Work out the finished part from the listing and answer in its coordinate system (mm). Face numbers are marked on the shaded views. A direction names the side the tool comes from. Round coordinates to 2 decimals unless told otherwise and drop trailing zeros. Loops run counter-clockwise (first coordinate to the right, second up) from the corner with the lowest first, then second, coordinate; pieces in that order, holes last.
```python
from build123d import *

# Parameters (mm, degrees)
BOSS_EXTRUDE1_DEPTH     = 27.94
CUT_EXTRUDE1_DEPTH      = 48.739163168
CUT_EXTRUDE1_DEPTH_BACK = 48.739163168
SKETCH3_R               = 6.35
CUT_EXTRUDE2_DEPTH      = 48.73916328
CUT_EXTRUDE2_DEPTH_BACK = 24.13
SKETCH4_R               = 8.001
CUT_EXTRUDE3_REACH      = 61.268
CUT_EXTRUDE3_START      = 12.192
SKETCH5_W               = 45.72
SKETCH5_H               = 20.574
SKETCH6_W               = 10.668
SKETCH6_H               = 4.572
CUT_EXTRUDE4_DEPTH      = 2.54
SKETCH7_W               = 12.7
SKETCH7_H               = 11.938
CUT_EXTRUDE5_DEPTH      = 2.54
FILLET1_R               = 5.08
CUT_EXTRUDE6_START      = 3.048
SKETCH8_W               = 48.26
SKETCH8_H               = 23.114
CUT_EXTRUDE6_DEPTH      = 12.7


with BuildPart() as part:
    # Sketch2 → Boss-Extrude1 (new body)
    with BuildSketch(Plane.XY):
        with BuildLine():
            Line((29.21, -5.08), (29.21, -25.4))
            Line((29.21, -25.4), (19.431, -25.4))
            ThreePointArc((19.431, -25.4), (10.16, -16.129), (0.889, -25.4))
            Line((0.889, -25.4), (-0.889, -25.4))
            ThreePointArc((-0.889, -25.4), (-10.16, -16.129), (-19.431, -25.4))
            Line((-19.431, -25.4), (-29.21, -25.4))
            Line((-29.21, -25.4), (-29.21, -5.08))
            ThreePointArc((-29.21, -5.08), (-27.722102448, -1.487897552), (-24.13, 0))
            Line((-24.13, 0), (24.13, 0))
            ThreePointArc((24.13, 0), (27.722102448, -1.487897552), (29.21, -5.08))
        make_face()
    extrude(amount=BOSS_EXTRUDE1_DEPTH)

    # Sketch3 → Cut-Extrude1 (cut, two sides: drawn at the far end of the back side and taken through both)
    with BuildSketch(Plane.XZ.offset(25.4).offset(-CUT_EXTRUDE1_DEPTH_BACK)):
        with Locations(Location((-12.954, 13.97, 0), (0, 0, 270))):
            Circle(SKETCH3_R)
        with Locations(Location((12.954, 13.97, 0), (0, 0, 270))):
            Circle(SKETCH3_R)
    extrude(amount=CUT_EXTRUDE1_DEPTH + CUT_EXTRUDE1_DEPTH_BACK, mode=Mode.SUBTRACT)

    # Sketch4 → Cut-Extrude2 (cut, two sides: drawn at the far end of the back side and taken through both)
    with BuildSketch(Plane.XZ.offset(25.4).offset(-CUT_EXTRUDE2_DEPTH_BACK)):
        with Locations(Location((-12.954, 13.97, 0), (0, 0, 215.950567609))):
            Circle(SKETCH4_R)
        with Locations(Location((12.954, 13.97, 0), (0, 0, 324.04943238))):
            Circle(SKETCH4_R)
    extrude(amount=CUT_EXTRUDE2_DEPTH + CUT_EXTRUDE2_DEPTH_BACK, mode=Mode.SUBTRACT)

    # Cut-Extrude3: up to this face of the body (flat: up to its plane)
    cut_extrude3_end = Plane(part.part.faces().sort_by_distance((-24.47856499, -25.4, 13.97))[0])
    # Sketch5 → Cut-Extrude3 (cut, up to the picked face)
    with BuildSketch(Plane.XZ.offset(1.27).offset(CUT_EXTRUDE3_START), mode=Mode.PRIVATE) as cut_extrude3_sk1:
        with Locations((0, 13.97)):
            Rectangle(SKETCH5_W, SKETCH5_H)
    cut_extrude3_tool1 = split(extrude(cut_extrude3_sk1.sketch, amount=CUT_EXTRUDE3_REACH, mode=Mode.PRIVATE), bisect_by=cut_extrude3_end, keep=Keep.BOTH, mode=Mode.PRIVATE)
    add(cut_extrude3_tool1.solids().sort_by(Axis((0, -13.462, 13.97), (0, -1, 0)))[0], mode=Mode.SUBTRACT)

    # Sketch6 → Cut-Extrude4 (cut)
    with BuildSketch(Plane.XZ.offset(13.462)):
        with Locations((0, 21.971)):
            Rectangle(SKETCH6_W, SKETCH6_H)
    cut_extrude4 = extrude(amount=-CUT_EXTRUDE4_DEPTH, mode=Mode.SUBTRACT)

    # Mirror1: Cut-Extrude4 across plane
    add(cut_extrude4.mirror(Plane.XY.offset(13.97)), mode=Mode.SUBTRACT)

    # Sketch7 → Cut-Extrude5 (cut)
    with BuildSketch(Plane(origin=(0, 0, 0), x_dir=(-1, 0, 0), z_dir=(0, 0, -1))):
        with Locations((0, -19.431)):
            Rectangle(SKETCH7_W, SKETCH7_H)
    extrude(amount=-CUT_EXTRUDE5_DEPTH, mode=Mode.SUBTRACT)

    # Fillet1
    fillet1_edges = [part.edges().sort_by_distance(p)[0] for p in [
        (-29.21, -15.24, 0),
        (-27.722102448, -1.487897552, 0),
        (0, 0, 0),
        (27.722102448, -1.487897552, 27.94),
        (27.722102448, -1.487897552, 0),
        (29.21, -15.24, 0),
        (0, 0, 27.94),
        (-27.722102448, -1.487897552, 27.94),
        (-29.21, -15.24, 27.94),
        (29.21, -15.24, 27.94),
    ]]
    fillet(fillet1_edges, radius=FILLET1_R)

    # Sketch8 → Cut-Extrude6 (cut)
    with BuildSketch(Plane.XZ.offset(13.462).offset(CUT_EXTRUDE6_START)):
        with Locations((0, 13.97)):
            Rectangle(SKETCH8_W, SKETCH8_H)
    extrude(amount=CUT_EXTRUDE6_DEPTH, mode=Mode.SUBTRACT)


solid = part.part
```
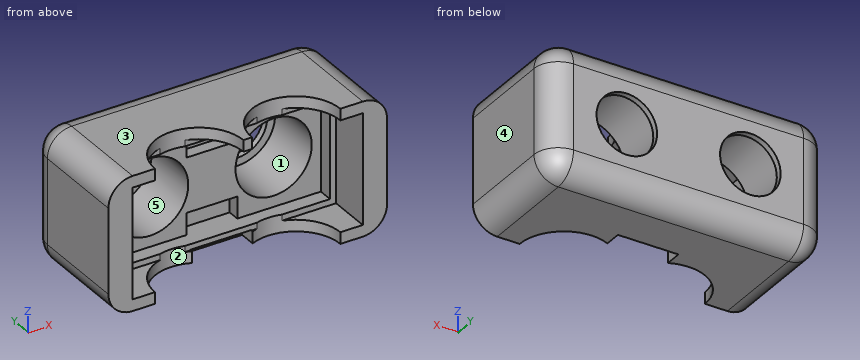
1. Find section B-B (x = -10.16). Write down the section's boundary in (y, z).
Answer key:
outline: (-16.13, 0) - (-5.08, 0) arc R5.08 ccw to (0, 5.08) - (0, 8.27) - (-1.27, 8.27) - (-1.27, 6.47) - (-13.46, 6.47) - (-13.46, 3.68) - (-16.13, 3.68) - close; (-16.13, 24.26) - (-13.46, 24.26) - (-13.46, 21.47) - (-1.27, 21.47) - (-1.27, 19.67) - (0, 19.67) - (0, 22.86) arc R5.08 ccw to (-5.08, 27.94) - (-16.13, 27.94) - close
2. Which of the six approach directions +Z, -Z, +X, -X, +Y, -Y give full straight-line access (tool end or side, diameter ignored) to the marked faces 1 and 2?
Answer key:
face 1: -Y
face 2: +Z, -Z, -Y
3. Find section C-C (y = -6). Write down the section's boundary in (x, z).
Answer key:
outline: (-29.21, 5.08) arc R5.08 ccw to (-24.13, 0) - (24.13, 0) arc R5.08 ccw to (29.21, 5.08) - (29.21, 22.86) arc R5.08 ccw to (24.13, 27.94) - (-24.13, 27.94) arc R5.08 ccw to (-29.21, 22.86) - close; hole circle Ø16 at (-12.95, 13.97); hole circle Ø16 at (12.95, 13.97)
4. Determine the mould class of the marked faces 3, 4 and 5 for opening direction X: +X half, -X half, draft (parallel to the pull), parting line (faces both ways), or undercut.
Answer key:
face 3: draft
face 4: +X half
face 5: undercut
5. Given pin 1 (3.5 mm diameter, centred on x = 17, z = 10, fed in from -Y); pin 2 (1.4 mm diameter, centred on x = 2, z = 6, fed in from -Y); pin 3 (10 mm diameter, centred on x = 16.5, y = -21, fed in from +Z); pin 4 (0.8 mm diameter, centred on y = -14.5, z = 2, fed in from -X), each flat-ended and moving along its own axis, determine where each tip first touches the part or whether it passes through.
Answer key:
pin 1: stops at y = -1.27
pin 2: stops at y = -10.92
pin 3: stops at z = 27.94
pin 4: stops at x = -28.45
6. Find section D-D (y = -23). Write down the section's boundary in (x, z), then the cut area to 3 significant figures.
Answer key:
outline: (-29.21, 5.08) arc R5.08 ccw to (-24.13, 0) - (-19.11, 0) - (-19.11, 2.41) - (-24.13, 2.41) - (-24.13, 25.53) - (-19.11, 25.53) - (-19.11, 27.94) - (-24.13, 27.94) arc R5.08 ccw to (-29.21, 22.86) - close; (-1.21, 25.53) - (1.21, 25.53) - (1.21, 27.94) - (-1.21, 27.94) - close; (19.11, 0) - (24.13, 0) arc R5.08 ccw to (29.21, 5.08) - (29.21, 22.86) arc R5.08 ccw to (24.13, 27.94) - (19.11, 27.94) - (19.11, 25.53) - (24.13, 25.53) - (24.13, 2.41) - (19.11, 2.41) - close
area: 316 mm2
7. Consider probe 1 along Z at (x, y) = (4.5, -12.5) (3 decimals); probe 2 along X at (y, z) = (-15, 15.75); probe 3 along X at (y, z) = (-6, 13.97) (3 decimals). Determine where each line is inside the solid, lowest interval first.
Answer key:
probe 1: z = 0 to 3.683, 8.255 to 19.685, 24.257 to 27.94
probe 2: x = -29.21 to -22.86, 22.86 to 29.21
probe 3: x = -29.21 to -20.955, -4.953 to 4.953, 20.955 to 29.21
8. Find section A-A (z = 13.97). Give the number of separate pieces and of enclosed holes in the cut face, then the cut area to 3 significant figures.
Answer key:
separate pieces: 3
enclosed holes: 0
area: 482 mm2
